The model under review builds one solid part; all positions refer to its coordinate system, in mm. Give positions to 0.01 mm unless a question says otherwise; leave off trailing zeros. Order: outer loops, then holes, each group sorted by start corner. A loop starts at its lowest first (then second) coordinate and runs counter-clockwise, first axis right, second up. Notation, with made-up numbers: (-16, 81) -> (-1, 81) arc R11 ccw to (-1, 102) -> close; hole circle Ø5 at (12.5, 21). An arc over 180 degrees is marked (long way). Use one line per item in the form item = value.
```python
from build123d import *

# Parameters (mm, degrees)
CYLINDER004_R     = 1.35
CYLINDER004_DEPTH = 2
CYLINDER003_R     = 0.75
CYLINDER003_DEPTH = 2
CYLINDER002_R     = 0.75
CYLINDER002_DEPTH = 2
CYLINDER001_R     = 0.97
CYLINDER001_DEPTH = 2
CYLINDER_R        = 2.75
CYLINDER_DEPTH    = 0.5
BOX_W             = 7
BOX_H             = 51.5
BOX_DEPTH         = 2


with BuildPart() as cylinder004:
    # Cylinder004 → Cylinder004 (new body)
    with BuildSketch(Plane(origin=(3.5, 2.35, 0), x_dir=(1, 0, 0), z_dir=(0, 0, 1))):
        Circle(CYLINDER004_R)
    extrude(amount=CYLINDER004_DEPTH)


with BuildPart() as cylinder003:
    # Cylinder003 → Cylinder003 (new body)
    with BuildSketch(Plane(origin=(3.5, 29, 0), x_dir=(1, 0, 0), z_dir=(0, 0, 1))):
        Circle(CYLINDER003_R)
    extrude(amount=CYLINDER003_DEPTH)


with BuildPart() as cylinder002:
    # Cylinder002 → Cylinder002 (new body)
    with BuildSketch(Plane(origin=(3.5, 50, 0), x_dir=(1, 0, 0), z_dir=(0, 0, 1))):
        Circle(CYLINDER002_R)
    extrude(amount=CYLINDER002_DEPTH)


with BuildPart() as cylinder001:
    # Cylinder001 → Cylinder001 (new body)
    with BuildSketch(Plane(origin=(3.5, 45.5, 0), x_dir=(1, 0, 0), z_dir=(0, 0, 1))):
        Circle(CYLINDER001_R)
    extrude(amount=CYLINDER001_DEPTH)


with BuildPart() as cylinder:
    # Cylinder → Cylinder (new body)
    with BuildSketch(Plane(origin=(3.5, 45.5, 1.5), x_dir=(1, 0, 0), z_dir=(0, 0, 1))):
        Circle(CYLINDER_R)
    extrude(amount=CYLINDER_DEPTH)


with BuildPart() as cut004:
    # Box → Box (new body)
    with BuildSketch(Plane.XY):
        with Locations((3.5, 25.75)):
            Rectangle(BOX_W, BOX_H)
    extrude(amount=BOX_DEPTH)

    # Cut: cut Cylinder
    add(cylinder.part, mode=Mode.SUBTRACT)

    # Cut001: cut Cylinder001
    add(cylinder001.part, mode=Mode.SUBTRACT)

    # Cut002: cut Cylinder002
    add(cylinder002.part, mode=Mode.SUBTRACT)

    # Cut003: cut Cylinder003
    add(cylinder003.part, mode=Mode.SUBTRACT)

    # Cut004: cut Cylinder004
    add(cylinder004.part, mode=Mode.SUBTRACT)


solid = cut004.part
```
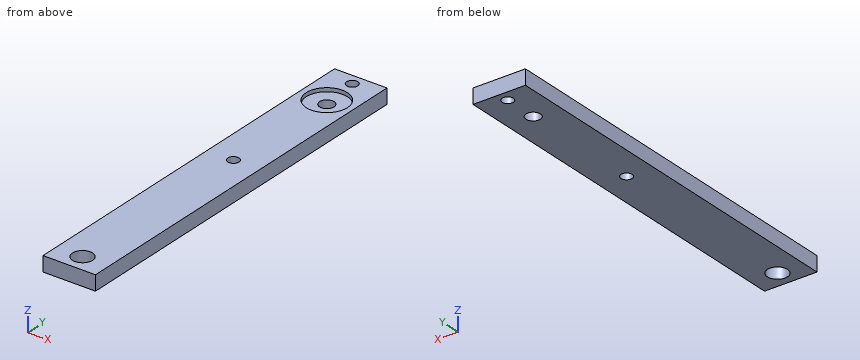
1. Add section C-C on z = 0.6. Give the boundary of the cut face in (x, y), then the cut area to 3 significant figures.
Values:
outline = (0, 0) -> (7, 0) -> (7, 51.5) -> (0, 51.5) -> close; hole circle Ø2.7 at (3.5, 2.35); hole circle Ø1.94 at (3.5, 45.5); hole circle Ø1.5 at (3.5, 29); hole circle Ø1.5 at (3.5, 50)
area = 348 mm^2
2. Add section A-A on y = 2.35. Give the boundary of the cut face in (x, z).
Values:
outline = (0, 0) -> (2.15, 0) -> (2.15, 2) -> (0, 2) -> close; (4.85, 0) -> (7, 0) -> (7, 2) -> (4.85, 2) -> close
3. For L1, parallel to Y at x = 3.5, z = 1.75; L2, parallel to Y at x = 3.5, z = 1.45; L3, parallel to X at y = 44.5, z = 1.8, list the stretches that pass through material, from the lowest coordinate up.
Values:
L1 = 0 to 1, 3.7 to 28.25, 29.75 to 42.75, 48.25 to 49.25, 50.75 to 51.5
L2 = 0 to 1, 3.7 to 28.25, 29.75 to 44.53, 46.47 to 49.25, 50.75 to 51.5
L3 = 0 to 0.94, 6.06 to 7
4. Add section B-B on x = 3.5. Give the boundary of the cut face in (y, z).
Values:
outline = (0, 0) -> (1, 0) -> (1, 2) -> (0, 2) -> close; (3.7, 0) -> (28.25, 0) -> (28.25, 2) -> (3.7, 2) -> close; (29.75, 0) -> (44.53, 0) -> (44.53, 1.5) -> (42.75, 1.5) -> (42.75, 2) -> (29.75, 2) -> close; (46.47, 0) -> (49.25, 0) -> (49.25, 2) -> (48.25, 2) -> (48.25, 1.5) -> (46.47, 1.5) -> close; (50.75, 0) -> (51.5, 0) -> (51.5, 2) -> (50.75, 2) -> close
5. Add section D-D on y = 45.5. Give the boundary of the cut face in (x, z), then the cut area to 3 significant figures.
Values:
outline = (0, 0) -> (2.53, 0) -> (2.53, 1.5) -> (0.75, 1.5) -> (0.75, 2) -> (0, 2) -> close; (4.47, 0) -> (7, 0) -> (7, 2) -> (6.25, 2) -> (6.25, 1.5) -> (4.47, 1.5) -> close
area = 8.34 mm^2
